```python
from build123d import *

# Parameters (mm, degrees)
SKETCH1_R           = 6.5
SKETCH1_R_2         = 2.5
BOSS_EXTRUDE1_DEPTH = 14
SKETCH2_W           = 7
SKETCH2_H           = 4.416086924
FILLET2_R           = 0.2
SKETCH4_R           = 2
CUT_EXTRUDE1_DEPTH  = 6


with BuildPart() as part:
    # Sketch1 → Boss-Extrude1 (new body)
    with BuildSketch(Plane.XY):
        Circle(SKETCH1_R)
        Circle(SKETCH1_R_2, mode=Mode.SUBTRACT)
    extrude(amount=BOSS_EXTRUDE1_DEPTH)

    # Sketch2 → Cut-Revolve1 (revolve, cut)
    with BuildSketch(Plane(origin=(0, 0, 0), x_dir=(0, 0, -1), z_dir=(1, 0, 0)), mode=Mode.PRIVATE) as cut_revolve1_sk:
        with Locations((-9.5, -7.008043462)):
            Rectangle(SKETCH2_W, SKETCH2_H)
    revolve(cut_revolve1_sk.sketch.rotate(Axis((0, 0, 15.643909914), (0, 0, -1)), 270), axis=Axis((0, 0, 15.643909914), (0, 0, -1)), mode=Mode.SUBTRACT)

    # Fillet2
    fillet2_edges = [part.edges().sort_by_distance(p)[0] for p in [
        (-6.5, 0, 13),
        (-6.5, 0, 6),
        (-6.5, 0, 0),
        (-6.5, 0, 14),
    ]]
    fillet(fillet2_edges, radius=FILLET2_R)

    # Sketch4 → Cut-Extrude1 (cut)
    with BuildSketch(Plane(origin=(6.5, 0, 0), x_dir=(0, 0, -1), z_dir=(1, 0, 0))):
        with Locations((-3, 0)):
            Circle(SKETCH4_R)
    extrude(amount=-CUT_EXTRUDE1_DEPTH, mode=Mode.SUBTRACT)


solid = part.part
```
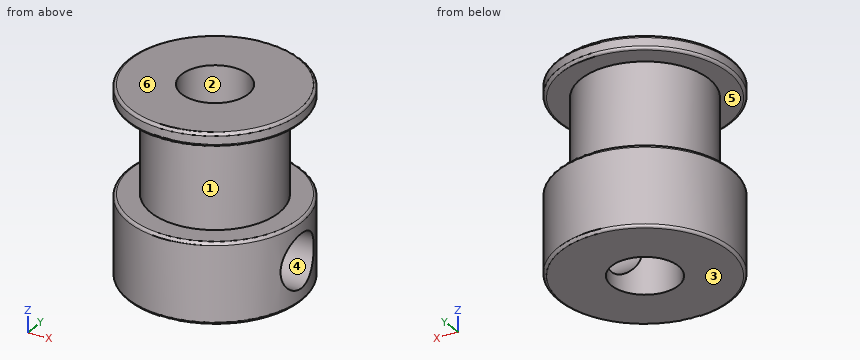
Work out the finished part from the listing and answer in its coordinate system (mm). Face numbers are marked on the shaded views. A direction names the side the tool comes from. Give positions to 0.01 mm unless a question says otherwise; leave off trailing zeros. Order: outer loops, then holes, each group sorted by start corner. A loop starts at its lowest first (then second) coordinate and runs counter-clockwise, first axis right, second up. Notation, with made-up numbers: M 46,-33.75 L 94,-33.75 A28 ccw 94,4.25 Z; hole C -21.5,4.25 d3. An arc over 180 degrees is marked long. Return JSON: item names as keys, results as strings.
1) Section C-C, the plane z = 5.25 is taken. Write down the section's boundary in (x, y).
Resolved:
{"outline": "C 0,0 d13; hole C 0,0 d5"}
2) Each of these flat-tipped pins is pushed along its axis until it touches: pin 1 (4 mm diameter, centred on x = 0, y = 0, fed in from +Z); pin 2 (5 mm diameter, centred on y = -3.5, z = 6, fed in from -X); pin 3 (5 mm diameter, centred on x = -3, z = 5, fed in from +Y); pin 4 (1.5 mm diameter, centred on x = 3.5, z = 8, fed in from -Y). Where does it stop, or does it pass through?
Resolved:
{"pin 1": "through", "pin 2": "x = -6.42", "pin 3": "y = 6.48", "pin 4": "y = -3.93"}
3) Section B-B, the plane x = 0 is taken. Write down the section's boundary in (y, z).
Resolved:
{"outline": "M -6.5,0.2 A0.2 ccw -6.3,0 L -2.5,0 L -2.5,14 L -6.3,14 A0.2 ccw -6.5,13.8 L -6.5,13.2 A0.2 ccw -6.3,13 L -4.8,13 L -4.8,6 L -6.3,6 A0.2 ccw -6.5,5.8 Z; M 2.5,0 L 6.3,0 A0.2 ccw 6.5,0.2 L 6.5,5.8 A0.2 ccw 6.3,6 L 4.8,6 L 4.8,13 L 6.3,13 A0.2 ccw 6.5,13.2 L 6.5,13.8 A0.2 ccw 6.3,14 L 2.5,14 Z"}
4) Section D-D, the plane x = 5 is taken. Give the number of separate pieces and of enclosed holes in the cut face, plus the area to 3 significant figures.
Resolved:
{"separate pieces": "2", "enclosed holes": "1", "area": "45.5 mm^2"}
5) Straight lines are drawn through the part: line 1 along Y through (x, z) = (0, 8); line 2 along Z through (x, y) = (0.25, 5.5); line 3 along Y through (x, z) = (0, 3.5). For each, find the intervals that lie inside material, in ascending order. Write a range as [from, to].
Resolved:
{"line 1": "[-4.8, -2.5], [2.5, 4.8]", "line 2": "[0, 6], [13, 14]", "line 3": "[-6.5, -2.5], [2.5, 6.5]"}
6) Section A-A, the plane y = 0 is taken. Write down the section's boundary in (x, z), plus the area to 3 significant figures.
Resolved:
{"outline": "M -6.5,0.2 A0.2 ccw -6.3,0 L -2.5,0 L -2.5,14 L -6.3,14 A0.2 ccw -6.5,13.8 L -6.5,13.2 A0.2 ccw -6.3,13 L -4.8,13 L -4.8,6 L -6.3,6 A0.2 ccw -6.5,5.8 Z; M 2.5,0 L 6.3,0 A0.2 ccw 6.5,0.2 L 6.5,1 L 2.5,1 Z; M 2.5,5 L 6.5,5 L 6.5,5.8 A0.2 ccw 6.3,6 L 4.8,6 L 4.8,13 L 6.3,13 A0.2 ccw 6.5,13.2 L 6.5,13.8 A0.2 ccw 6.3,14 L 2.5,14 Z", "area": "72.1 mm^2"}
7) For a pull along Y with two mould halves and no side action, classify the marked faces 1, 2 and 3 as +Y half, -Y half, draft (parallel to the pull), parting line (faces both ways), or undercut.
Resolved:
{"face 1": "parting line", "face 2": "undercut", "face 3": "draft"}
8) A tool of negligible diameter and unlimited length cuts with its end or side. For the marked faces 4, 5 and 6, from which of +Z, -Z, +X, -X, +Y, -Y can it reach the whole face along a straight path? Write none if from no direction.
Resolved:
{"face 4": "+X", "face 5": "none", "face 6": "+Z, +X, -X, +Y, -Y"}
